Part model, mm, in its own coordinate system. A direction names the side the tool comes from. Give positions to 0.01 mm unless a question says otherwise; leave off trailing zeros. Order: outer loops, then holes, each group sorted by start corner. A loop starts at its lowest first (then second) coordinate and runs counter-clockwise, first axis right, second up. Notation, with made-up numbers: (58.5, 33) -> (82.5, 33) arc R26 cw to (82.5, 64) -> close; hole circle Ø7 at (-0.75, 33). An arc over 180 degrees is marked (long way). Write item = value, one per line. Start each with the question number.
(1) Which spindle directions (+Z, -Z, +X, -X, +Y, -Y) get a long thin tool onto all of the face, cutting with end or side? Do faces 4 (the flat face through (-2, 0, 0)), 5 (the cylindrical face through (1.908, 0.687, 12.887)), 6 (the flat face through (-0.5, 0, 1)). Say none if no direction does.
(2) Two-plate mould, pull along X, no slides. Class faces 1 (the flat face through (0, 0, 1.9)), 2 (the conical face through (-3.78, 0.08, 0.13)), 3 (the flat face through (0, 0, 23.2)): pulls with the +X half, pulls with the -X half, needs draft (parallel to the pull), parting line crosses it, or undercut.
(3) Probe line 1 along Z through (x, y) = (1, 3); line 2 along Y through (x, z) = (0, 4.5); line 3 along X through (y, z) = (-1.5, 18.75). List the from-to ranges inside material, lowest first. Write a range as from..to.
(4) Saw through at B-B, the plane z = 14.75. List the corners of the cut face in (x, y).
(5) Flat gauge pins, fed straight in: pin 1 (1.5 mm diameter, centred on y = 0, z = 15, fed in from -X); pin 2 (3 mm diameter, centred on x = -1, z = 12, fed in from +Y); pin 3 (3 mm diameter, centred on y = -2, z = 18, fed in from -X). Where does each tip first touch, or does it go through?
(6) Saw through at A-A, the plane x = 0. List the corners of the cut face in (y, z), then the cut area to 3 significant figures.
from build123d import *

# Parameters (mm, degrees)
SKETCH_1_R          = 4
EXTRUDE_1_DEPTH     = 3.2
SKETCH_2_R          = 2
EXTRUDE_2_DEPTH     = 20
CUT_EXTRUDE_1_DEPTH = 1.9
CHAMFER_1_SIZE      = 0.35


with BuildPart() as part:
    # Эскиз1 → Вытянуть1 (new body)
    with BuildSketch(Plane.XY):
        with Locations(Location((0, 0, 0), (0, 0, 97.180755781))):
            Circle(SKETCH_1_R)
    extrude(amount=EXTRUDE_1_DEPTH)

    # Эскиз2 → Вытянуть2 (add)
    with BuildSketch(Plane.XY.offset(3.2)):
        with Locations((0, 0.08601646)):
            Circle(SKETCH_2_R)
    extrude(amount=EXTRUDE_2_DEPTH)

    # Эскиз3 → Вырез-Вытянуть1 (cut)
    with BuildSketch(Plane(origin=(0, 0, 0), x_dir=(-1, 0, 0), z_dir=(0, 0, -1))):
        Polygon((0.5, 4.203337699), (0.5, -4.490059234), (-0.5, -4.7079676), (-0.5, 4.570341264), align=None)
    extrude(amount=-CUT_EXTRUDE_1_DEPTH, mode=Mode.SUBTRACT)

    # Фаска1
    chamfer_1_edges = [part.edges().sort_by_distance(p)[0] for p in [
        (-4, 0, 0),
        (4, 0, 0),
        (-2, 0.08601646, 23.2),
    ]]
    chamfer(chamfer_1_edges, length=CHAMFER_1_SIZE)


solid = part.part
Results list:
q1.face_4 = -Z, +X, -X, +Y, -Y
q1.face_5 = +Z
q1.face_6 = -Z, +Y, -Y
q2.face_1 = undercut
q2.face_2 = pulls with the -X half
q2.face_3 = needs draft
q3.line_1 = 0..3.2
q3.line_2 = -1.91..2.09
q3.line_3 = -1.22..1.22
q4.outline = circle Ø4 at (0, 0.09)
q5.pin_1 = -2
q5.pin_2 = 2.09
q5.pin_3 = -1.91
q6.outline = (-4, 1.9) -> (4, 1.9) -> (4, 3.2) -> (2.09, 3.2) -> (2.09, 22.85) -> (1.74, 23.2) -> (-1.56, 23.2) -> (-1.91, 22.85) -> (-1.91, 3.2) -> (-4, 3.2) -> close
q6.area = 90.3 mm^2
